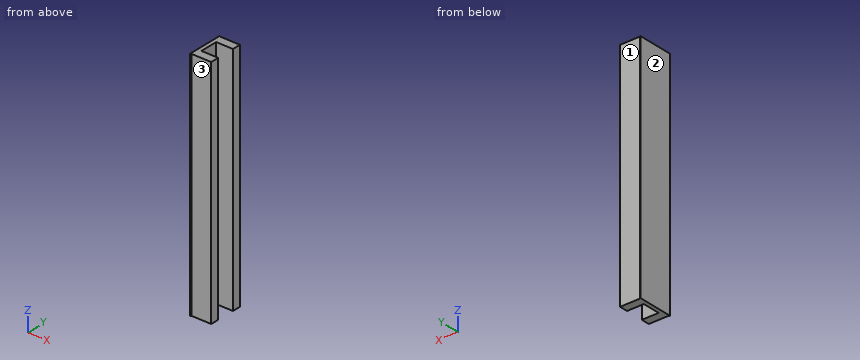
Autodesk Inventor part; units mm, degrees
ref_plane "YZ Plane" through (0, 0, 0) normal (1, 0, 0) x (0, 1, 0)
ref_plane "XZ Plane" through (0, 0, 0) normal (0, 1, 0) x (-1, 0, 0)
ref_plane "XY Plane" through (0, 0, 0) normal (0, 0, 1) x (1, 0, 0)
sketch "Sketch1" plane through (0, 0, 0) normal (0, 1, 0) x (-1, 0, 0)
  line L0 (0, 279.3478) -> (-39.1304, 279.3478)
  line L1 (-39.1304, 279.3478) -> (-39.1304, -195.6522)
  line L2 (-39.1304, -195.6522) -> (0, -195.6522)
  line L3 (0, -195.6522) -> (0, 279.3478)
  line L4 (-39.1304, 279.3478) -> (-29.1304, 279.3478)
  line L5 (-29.1304, 254.3478) -> (-39.1304, 254.3478)
  line L6 (-39.1304, 254.3478) -> (-39.1304, 279.3478)
  line L7 (-39.1304, -195.6522) -> (-29.1304, -195.6522)
  line L8 (-29.1304, -170.6522) -> (-39.1304, -170.6522)
  line L9 (-39.1304, -170.6522) -> (-39.1304, -195.6522)
  point P0 (0, 0)
  point P1 (-39.1304, 254.3478)
  dimension "d0" = 475
  dimension "d4" = 25
  dimension "d5" = 25
extrude "Extrusion1" add sketch "Sketch1" along normal blind 160
sketch "Sketch2" plane through (0, 0, 279.3478) normal (0, 0, 1) x (1, 0, 0)
  line L0 (0, 160) -> (39.1304, 160)
  line L1 (0, 160) -> (39.1304, 160)
  line L2 (39.1304, 160) -> (39.1304, 0)
  line L3 (39.1304, 0) -> (0, 0)
  line L4 (0, 0) -> (0, 160)
  line L5 (39.1304, 160) -> (29.1304, 160)
  line L6 (29.1304, 160) -> (29.1304, 115)
  line L7 (29.1304, 115) -> (39.1304, 115)
  line L8 (39.1304, 115) -> (39.1304, 160)
  line L9 (39.1304, 0) -> (29.1304, 0)
  line L10 (29.1304, 0) -> (29.1304, 45)
  line L11 (29.1304, 45) -> (39.1304, 45)
  line L12 (39.1304, 45) -> (39.1304, 0)
  circle A0 centre (39.1304, 80) radius 18
  line L13 (35.1304, 75) -> (39.1304, 75)
  line L14 (39.1304, 75) -> (39.1304, 98)
  line L15 (39.1304, 98) -> (35.1304, 98)
  line L16 (35.1304, 98) -> (35.1304, 75)
  line L17 (35.1304, 75) -> (39.1304, 75)
  line L18 (39.1304, 75) -> (39.1304, 62)
  line L19 (39.1304, 62) -> (35.1304, 62)
  line L20 (35.1304, 62) -> (35.1304, 75)
  line L21 (39.1304, 0) -> (39.1304, 160)
  line L22 (0, 160) -> (19.1304, 160)
  line L23 (19.1304, 160) -> (19.1304, 0)
  line L24 (19.1304, 0) -> (0, 0)
  line L25 (0, 0) -> (0, 160)
  point P0 (0, 0)
  point P1 (34.1304, 115)
  point P2 (34.1304, 160)
  point P3 (39.1304, 45)
  point P4 (39.1304, 115)
  dimension "d6" = 10
  dimension "d7" = 45
  dimension "d8" = 45
  dimension "d9" = 4
  dimension "d10" = 36
  dimension "d11" = 80
  dimension "d12" = 80
  dimension "d15" = 20
extrude "Extrusion2" cut sketch "Sketch2" against normal up to surface (475 mm away) contours L0 L23 L3 L4 | L0 L2 L7 L6 | L10 L11 L2 L3 | L2 L13 L16 A0 | A0 L16 L15 | L2 A0 L20 L13 | L19 L20 A0
sketch "Sketch3" plane through (0, 160, 0) normal (0, 1, 0) x (1, 0, 0)
  line L0 (-18, 349) -> (160, 349)
  line L1 (160, 349) -> (160, 190.6522)
  line L2 (160, 190.6522) -> (-18, 190.6522)
  line L3 (-18, 190.6522) -> (-18, 349)
  line L4 (19.1304, -279.3478) -> (29.1304, -279.3478)
  point P0 (0, 0)
  dimension "d16" = 470
extrude "Extrusion3" cut sketch "Sketch3" against normal blind 200
sketch "Sketch4" plane through (39.1304, 98, 279.3478) normal (1, 0, 0) x (0, 0, -1)
  line L0 (470, 0) -> (470, 17)
  line L1 (470, 17) -> (0, 17)
  line L2 (0, 0) -> (0, 17)
  line L3 (0, 0) -> (470, 0)
  line L4 (470, -53) -> (470, -36)
  line L5 (470, -36) -> (0, -36)
  line L6 (0, -53) -> (0, -36)
  line L7 (0, -53) -> (470, -53)
  point P0 (279.3478, -98)
extrude "Extrusion4" add sketch "Sketch4" along normal blind 30
sketch "Sketch5" plane through (19.1304, 0, 279.3478) normal (-1, 0, 0) x (0, 0, 1)
  line L0 (-470, 160) -> (-470, 0)
  line L1 (0, 0) -> (-470, 0)
  line L2 (0, 160) -> (0, 0)
  line L3 (-470, 160) -> (0, 160)
  point P0 (-279.3478, 0)
extrude "Extrusion5" add sketch "Sketch5" along normal blind 5
sketch "Sketch6" plane through (29.1304, 115, 279.3478) normal (0, 0, 1) x (1, 0, 0)
  line L0 (9, 13) -> (-3, 13)
  line L1 (-3, 13) -> (-3, 45)
  line L2 (-3, 45) -> (9, 45)
  line L3 (9, 45) -> (9, 13)
  line L4 (-15, -115) -> (0, -115)
  line L5 (11, -83) -> (-3, -83)
  line L6 (-3, -83) -> (-3, -115)
  line L7 (-3, -115) -> (11, -115)
  line L8 (11, -115) -> (11, -83)
  line L9 (0, -70) -> (40, -70)
  line L10 (0, 0) -> (40, 0)
  line L11 (0, 0) -> (0, 45)
  point P0 (-29.1304, -115)
  point P1 (0, -115)
  dimension "d23" = 13
  dimension "d24" = 13
  dimension "d25" = 3
extrude "Extrusion6" cut sketch "Sketch6" against normal blind 500
sketch "Sketch7" plane through (35.1304, 62, 279.3478) normal (0, 0, 1) x (1, 0, 0)
  line L0 (55, 54) -> (-8, 54)
  line L1 (-8, 54) -> (-8, -18)
  line L2 (-8, -18) -> (55, -18)
  line L3 (55, -18) -> (55, 54)
  line L4 (-6, 53) -> (34, 53)
  line L5 (-6, -17) -> (34, -17)
  line L6 (-6, -30) -> (-6, -17)
  line L7 (-9, 98) -> (-21, 98)
  line L8 (-21, 98) -> (63, 98)
  line L9 (63, 98) -> (63, -62)
  line L10 (63, -62) -> (-21, -62)
  line L11 (-21, -62) -> (-21, 98)
  point P0 (-35.1304, -62)
  point P1 (-9, 98)
  dimension "d28" = 1
  dimension "d29" = 1
  dimension "d30" = 2
extrude "Extrusion7" cut sketch "Sketch7" against normal blind 1000
properties part number "MainRails" material "Aluminum 6061"
CAD build for the part. Positions are in the model's coordinates, mm. Face numbers are marked on the shaded views. A direction names the side the tool comes from. Round coordinates to 2 decimals unless told otherwise and drop trailing zeros. Order: outer loops, then holes, each group sorted by start corner. A loop starts at its lowest first (then second) coordinate and runs counter-clockwise, first axis right, second up.
Q1. Which spindle directions (+Z, -Z, +X, -X, +Y, -Y) get a long thin tool onto all of the face, cutting with end or side? Do the marked faces 1, 2 and 3. Say none if no direction does.
Q2. Slice it at B-B (z = 18). Write the cut outline in (x, y).
Q3. Slice it at A-A (x = 42.5). Write the cut outline in (y, z).
Q4. Slice it at C-C (y = 88.5). Write the cut outline in (x, z), and give its area (3 significant figures).
Q5. Wall check: L1, parallel to Y at x = 36, z = -56; L2, parallel to Y at x = 30, z = 10; L3, parallel to X at y = 74.5, z = 133. Give the ranges that are in metal, low to high.
Q6. Drop flat-ended pins along their axis: pin 1 (3 mm diameter, centred on y = 65, z = 122, fed in from +X); pin 2 (17 mm diameter, centred on x = 48.5, z = 4.5, fed in from +Y); pin 3 (0.5 mm diameter, centred on y = 44.5, z = 44.5, fed in from +X); pin 4 (10 mm diameter, centred on x = 63.5, y = 71.5, fed in from +Z). Give the stop position or say it passes through.
Results below:
1. face 1: +Z, -Z, +X, +Y
1. face 2: +Z, -Z, -X, +Y, -Y
1. face 3: +Z, -Z, +X, -Y
2. outline: (27.13, 44) - (29.13, 44) - (29.13, 45) - (69.13, 45) - (69.13, 62) - (35.13, 62) - (35.13, 98) - (69.13, 98) - (69.13, 115) - (29.13, 115) - (29.13, 116) - (27.13, 116) - close
3. outline: (45, -190.65) - (62, -190.65) - (62, 279.35) - (45, 279.35) - close; (98, -190.65) - (115, -190.65) - (115, 279.35) - (98, 279.35) - close
4. outline: (27.13, -190.65) - (35.13, -190.65) - (35.13, 279.35) - (27.13, 279.35) - close
4. area: 3,760 mm2
5. L1: y = 45 to 62, 98 to 115
5. L2: y = 45 to 115
5. L3: x = 27.13 to 35.13
6. pin 1: stops at x = 35.13
6. pin 2: stops at y = 115
6. pin 3: stops at x = 29.13
6. pin 4: passes through
